Here's the drawing with two shaded views (mm, measured from the low corner). I have some questions. A direction names the side the tool comes from. Coordinates: 2 decimals unless noted, no trailing zeros. Write each loop counter-clockwise with the first axis right and the second up, starting at its lowest first coordinate (ties: lowest second). Pieces come first, ordered by that corner, then holes.
Item 1: We'd pull the mould along Z, two halves only. Please class the marked faces 1, 2 and 3: +Z half, -Z half, draft (parallel to the pull), parting line (faces both ways), or undercut.
Item 2: If we section it at B-B (x = 29): Please give me the cut outline in (y, z).
Item 3: I'm going to push flat-ended pins straight in: pin 1 Ø20.5 at (x, y) = (26.5, 35.5) entering from +Z; pin 2 Ø3.5 at (x, z) = (9, 7.5) entering from +Y; pin 3 Ø1 at (y, z) = (44.5, 0.5) entering from -X. Where does each tip first touch, or does it pass through?
Item 4: If I drill on line 1 (Y direction, x = 19, z = 1.2); line 2 (Y direction, x = 29, z = 0.75); line 3 (Z direction, x = 23.5, y = 22), over which ranges is the centre line in solid material (lowest first)?
Item 5: If we section it at C-C (y = 6): Please give me the cut outline in (x, z), then the cut area to 3 significant figures.
Item 6: If we section it at D-D (z = 9): Please give me the cut outline in (x, y), then the cut area to 3 significant figures.
Item 7: If we section it at A-A (y = 18): Please give me the cut outline in (x, z).
Item 8: For the marked faces 4, 5, 6 and 7, which set-ups out of +Z, -Z, +X, -X, +Y, -Y let a thin tool reach every point of the face, with its end or its side?
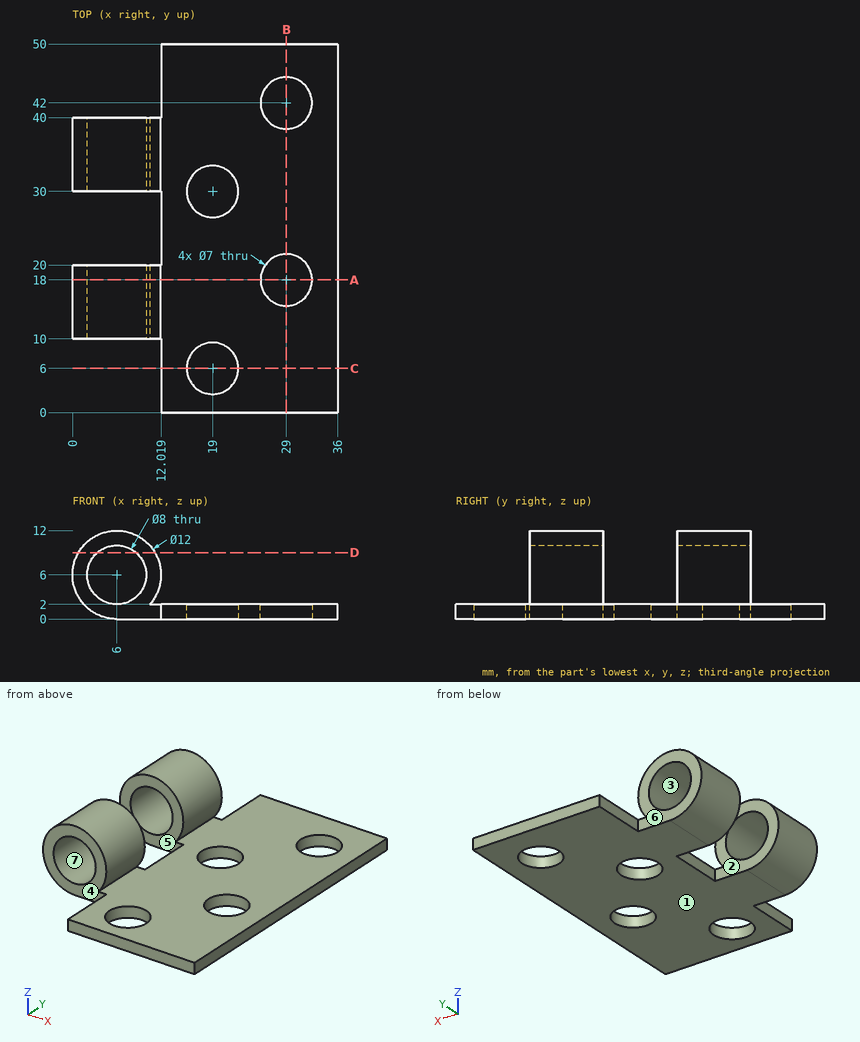
Answer list:
1. face 1: -Z half
1. face 2: draft
1. face 3: undercut
2. outline: (0, 0) - (14.5, 0) - (14.5, 2) - (0, 2) - close; (21.5, 0) - (38.5, 0) - (38.5, 2) - (21.5, 2) - close; (45.5, 0) - (50, 0) - (50, 2) - (45.5, 2) - close
3. pin 1: stops at z = 2
3. pin 2: stops at y = 40
3. pin 3: stops at x = 12.02
4. line 1: y = 0 to 2.5, 9.5 to 26.5, 33.5 to 50
4. line 2: y = 0 to 14.5, 21.5 to 38.5, 45.5 to 50
4. line 3: z = 0 to 2
5. outline: (12.02, 0) - (15.5, 0) - (15.5, 2) - (12.02, 2) - close; (22.5, 0) - (36, 0) - (36, 2) - (22.5, 2) - close
5. area: 34.0 mm2
6. outline: (0.8, 10) - (3.35, 10) - (3.35, 20) - (0.8, 20) - close; (0.8, 30) - (3.35, 30) - (3.35, 40) - (0.8, 40) - close; (8.65, 10) - (11.2, 10) - (11.2, 20) - (8.65, 20) - close; (8.65, 30) - (11.2, 30) - (11.2, 40) - (8.65, 40) - close
6. area: 102 mm2
7. outline: (6, 0) - (25.5, 0) - (25.5, 2) - (10.47, 2) arc R6 ccw (long way) to start; (32.5, 0) - (36, 0) - (36, 2) - (32.5, 2) - close; hole circle Ø8 at (6, 6)
8. face 4: +Z, -Z, -X, -Y
8. face 5: +Z, -Z, -X
8. face 6: +Z, -Z, -X, +Y
8. face 7: +Y, -Y
